Source: CAD feature listing. Evaluate the final solid. Frame: model axes, mm. Face numbers are marked on the shaded views. Round coordinates to 2 decimals unless told otherwise and drop trailing zeros. Loops run counter-clockwise (first coordinate to the right, second up) from the corner with the lowest first, then second, coordinate; pieces in that order, holes last. Notation, with made-up numbers: M 61,-17 L 88,-17 A16 ccw 88,1 Z; hole C 25.25,33 d7. An arc over 180 degrees is marked long. Answer as a JSON object with one key per item and string values.
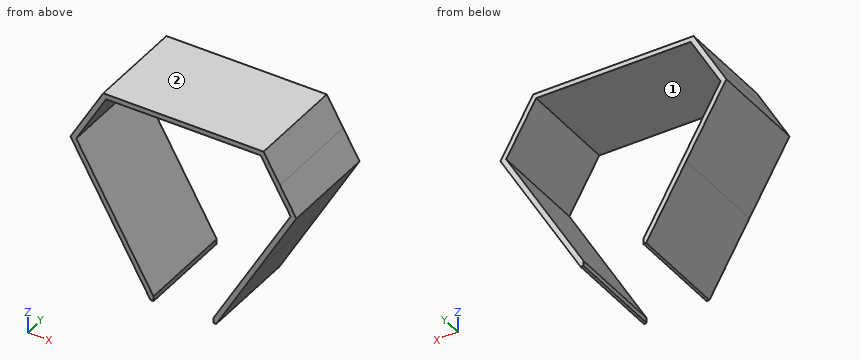
Autodesk Inventor part; units mm, degrees
ref_plane "YZ Plane" through (0, 0, 0) normal (1, 0, 0) x (0, 1, 0)
ref_plane "XZ Plane" through (0, 0, 0) normal (0, 1, 0) x (-1, 0, 0)
ref_plane "XY Plane" through (0, 0, 0) normal (0, 0, 1) x (1, 0, 0)
sketch "スケッチ1" plane through (0, 0, 0) normal (0, 1, 0) x (-1, 0, 0)
  line L0 (137.5, 79.3857) -> (-137.5, 79.3857)
  line L1 (-137.5, 79.3857) -> (0, -158.7713)
  line L2 (0, -158.7713) -> (137.5, 79.3857)
  line L3 (137.5, 79.3857) -> (-68.75, -39.6928) construction
  line L4 (77.5, 79.3857) -> (107.5, 27.4241)
  line L5 (-107.5, 27.4241) -> (-77.5, 79.3857)
  line L6 (30, -106.8098) -> (-30, -106.8098)
  line L7 (80.3868, 84.3857) -> (0, 84.3857)
  line L8 (80.3868, 84.3857) -> (96.8301, 55.9049)
  line L9 (0, 0) -> (0, 84.3857) construction
  line L10 (-80.3868, 84.3857) -> (0, 84.3857)
  line L11 (-80.3868, 84.3857) -> (-96.8301, 55.9049)
  line L12 (-113.2735, 27.4241) -> (-96.8301, 55.9049)
  line L13 (-113.2735, 27.4241) -> (-73.0801, -42.1928)
  line L14 (-32.8868, -111.8098) -> (-73.0801, -42.1928)
  line L15 (-32.8868, -111.8098) -> (0, -111.8098)
  line L16 (32.8868, -111.8098) -> (0, -111.8098)
  line L17 (32.8868, -111.8098) -> (73.0801, -42.1928)
  line L18 (113.2735, 27.4241) -> (73.0801, -42.1928)
  line L19 (113.2735, 27.4241) -> (96.8301, 55.9049)
  line L20 (30, -111.8098) -> (30, -106.8098)
  line L21 (-30, -111.8098) -> (-30, -106.8098)
  line L22 (-30, -106.8098) -> (30, -106.8098)
  point P0 (-30, -106.8098)
  point P1 (-107.5, 27.4241)
  point P2 (-77.5, 79.3857)
  point P3 (30, -106.8098)
  dimension "d0" = 275
  dimension "d1" = 60
  dimension "d4" = 360
  dimension "d6" = 5
  dimension "d7" = 5
  dimension "d10" = 360
extrude "押し出し1" add sketch "スケッチ1" along normal blind 100 contours L0 L11 L10 L7 L8 | L0 L8 L19 L2 L4 | L5 L1 L12 L11 L0 | L2 L19 L18 L17 L16 L20 | L1 L21 L15 L14 L13 L12
properties part number "base_cover"
Item 1: Section D-D on x = -25. Return the cut outline in (y, z), then the cut area to 3 significant figures.
Answer sheet:
{"outline": "M 0,79.39 L 100,79.39 L 100,84.39 L 0,84.39 Z", "area": "500 mm²"}
Item 2: Section A-A on z = 16. Return the cut outline in (x, y), then the cut area to 3 significant figures.
Answer sheet:
{"outline": "M -106.68,0 L -100.9,0 L -100.9,100 L -106.68,100 Z; M 100.9,0 L 106.68,0 L 106.68,100 L 100.9,100 Z", "area": "1,150 mm²"}
Item 3: Pull-direction query (Z, two-part tool) for the marked faces 1 and 2; classes: pulls with the +Z half, pulls with the -Z half, needs draft (parallel to the pull), parting line crosses it, or undercut.
Answer sheet:
{"face 1": "undercut", "face 2": "pulls with the +Z half"}
Item 4: Section C-C on y = 77.5. Return the cut outline in (x, z).
Answer sheet:
{"outline": "M -113.27,27.42 L -73.08,-42.19 L -32.89,-111.81 L -30,-111.81 L -30,-106.81 L -107.5,27.42 L -77.5,79.39 L 77.5,79.39 L 107.5,27.42 L 30,-106.81 L 30,-111.81 L 32.89,-111.81 L 73.08,-42.19 L 113.27,27.42 L 96.83,55.9 L 80.39,84.39 L -80.39,84.39 L -96.83,55.9 Z"}
Item 5: Contact query for flat-ended pins moving along their axis: pin 1 Ø2.5 at (y, z) = (35, -110) entering from -X; pin 2 Ø3 at (x, y) = (-72.5, 75.5) entering from -Z; pin 3 Ø4 at (y, z) = (80, 28) entering from -X; pin 4 Ø4 at (y, z) = (88.5, 59.5) entering from +X. Output: stop coordinate, or through.
Answer sheet:
{"pin 1": "stops at x = -34.65", "pin 2": "stops at z = -45.8", "pin 3": "stops at x = -113.27", "pin 4": "stops at x = 95.91"}
Item 6: Section B-B on x = -53. Return the cut outline in (y, z).
Answer sheet:
{"outline": "M 0,-76.97 L 100,-76.97 L 100,-66.97 L 0,-66.97 Z; M 0,79.39 L 100,79.39 L 100,84.39 L 0,84.39 Z"}
Item 7: Line query: probe 1 along X at (y, z) = (17, -87.5); probe 2 along Z at (x, y) = (19.5, 83); probe 3 along Z at (x, y) = (38.5, 54.5). Output: solid intervals per line, ascending. Write a range as from..to.
Answer sheet:
{"probe 1": "x = -46.92..-41.15, 41.15..46.92", "probe 2": "z = 79.39..84.39", "probe 3": "z = -102.09..-92.09, 79.39..84.39"}
